```python
from build123d import *

# Parameters (mm, degrees)
SKETCH1_R                 = 6.35
BOSS_EXTRUDE1_DEPTH       = 2.9591
F_4_CLEARANCE_HOLE1_D     = 2.9464
F_4_CLEARANCE_HOLE1_DEPTH = 2.9591


with BuildPart() as part:
    # Sketch1 → Boss-Extrude1 (new body)
    with BuildSketch(Plane(origin=(0, 0, 0), x_dir=(1, 0, 0), z_dir=(0, 1, 0))):
        Polygon((6.35, 15.6591), (15.6591, 15.6591), (15.6591, 6.35), (12.7, 6.35), (12.7, -6.35), (15.6591, -6.35), (15.6591, -15.6591), (6.35, -15.6591), (6.35, -12.7), (-6.35, -12.7), (-6.35, -15.6591), (-15.6591, -15.6591), (-15.6591, -6.35), (-12.7, -6.35), (-12.7, 6.35), (-15.6591, 6.35), (-15.6591, 15.6591), (-6.35, 15.6591), (-6.35, 12.7), (6.35, 12.7), align=None)
        Circle(SKETCH1_R, mode=Mode.SUBTRACT)
    extrude(amount=BOSS_EXTRUDE1_DEPTH)

    # #4 Clearance Hole1
    with Locations(Plane(origin=(-7.797262335, 2.9591, -11.472083192), x_dir=(1, 0, 0), z_dir=(0, 1, 0))):
        with Locations((7.797262335, -1.947083192), (17.322262335, -11.472083192), (7.797262335, -20.997083192), (-1.727737665, -11.472083192)):
            Hole(F_4_CLEARANCE_HOLE1_D / 2, depth=F_4_CLEARANCE_HOLE1_DEPTH)


solid = part.part
```
Geometry check sheet. Reference: the model listing, model coordinates, mm. A direction names the side the tool comes from. Give positions to 0.01 mm unless a question says otherwise; leave off trailing zeros. Loops run counter-clockwise (first coordinate to the right, second up) from the corner with the lowest first, then second, coordinate; pieces in that order, holes last. Notation, with made-up numbers: M 30,1.5 L 63,1.5 A31 cw 63,38.5 Z; hole C -10,40.5 d9. An arc over 180 degrees is marked long. Write item = value, one per line. Start each with the question number.
1. Thickness scan on probe 1 along Z at (x, y) = (0, 1.75); probe 2 along X at (y, z) = (1.4, -14); probe 3 along X at (y, z) = (1.9, -0.5). Record the ranges inside material, lowest first.
2. Draft check along Z on faces 1 (the face through (-11, 1, 15.659)), 2 (the face through (-15.659, 1, -11)), 3 (the face through (0.192, 1.459, 8.064)). Enter one of: +Z half, -Z half, draft (parallel to the pull), parting line (faces both ways), or undercut.
3. Section check B-B, the plane z = 0. Enter the section's corners in (x, y), plus the area to 3 significant figures.
4. Section check D-D, the plane z = -5.5. Enter the section's corners in (x, y).
5. Go/stop test with flat-tipped pins: P1, Ø1.5, axis at y = 1, z = -5.5, coming from the -X side; P2, Ø1, axis at y = 1.5, z = -2, coming from the +X side; P3, Ø0.9, axis at x = -3, y = 1, coming from the +Z side. Record where each tip stops, or that it passes through.
6. Section check C-C, the plane x = -5. Enter the section's corners in (y, z).
7. Section check A-A, the plane x = 0. Enter the section's corners in (y, z).
8. Tool access check on faces 4 (the face through (-12.7, 1, 0)), 5 (the face through (14, 1, -6.35)), 6 (the face through (-6.35, 1, -14)), 7 (the face through (-6.35, 1, 14)), 8 (the face through (-15.659, 1, 11)). Record the directions out of +Z, -Z, +X, -X, +Y, -Y that give a thin tool (end or side, any length) a straight path to the whole face; none if there is none.
Values follow:
q1.probe_1 = -12.7 to -11, -8.05 to -6.35, 6.35 to 8.05, 11 to 12.7
q1.probe_2 = -15.66 to -6.35, 6.35 to 15.66
q1.probe_3 = -12.7 to -10.91, -8.14 to -6.33, 6.33 to 8.14, 10.91 to 12.7
q2.face_1 = +Z half
q2.face_2 = draft
q2.face_3 = undercut
q3.outline = M -12.7,0 L -11,0 L -11,2.96 L -12.7,2.96 Z; M -8.05,0 L -6.35,0 L -6.35,2.96 L -8.05,2.96 Z; M 6.35,0 L 8.05,0 L 8.05,2.96 L 6.35,2.96 Z; M 11,0 L 12.7,0 L 12.7,2.96 L 11,2.96 Z
q3.area = 20.1 mm^2
q4.outline = M -12.7,0 L -3.17,0 L -3.17,2.96 L -12.7,2.96 Z; M 3.17,0 L 12.7,0 L 12.7,2.96 L 3.17,2.96 Z
q5.P1 = -12.7
q5.P2 = 12.7
q5.P3 = 12.7
q6.outline = M 0,-12.7 L 2.96,-12.7 L 2.96,-3.91 L 0,-3.91 Z; M 0,3.91 L 2.96,3.91 L 2.96,12.7 L 0,12.7 Z
q7.outline = M 0,-12.7 L 2.96,-12.7 L 2.96,-11 L 0,-11 Z; M 0,-8.05 L 2.96,-8.05 L 2.96,-6.35 L 0,-6.35 Z; M 0,6.35 L 2.96,6.35 L 2.96,8.05 L 0,8.05 Z; M 0,11 L 2.96,11 L 2.96,12.7 L 0,12.7 Z
q8.face_4 = -X, +Y, -Y
q8.face_5 = +X, +Y, -Y
q8.face_6 = -Z, +Y, -Y
q8.face_7 = +Z, +Y, -Y
q8.face_8 = +Z, -Z, -X, +Y, -Y
